Source: CAD feature listing. Evaluate the final solid. Frame: model axes, mm. A direction names the side the tool comes from. Round coordinates to 2 decimals unless told otherwise and drop trailing zeros. Order: outer loops, then holes, each group sorted by start corner. A loop starts at its lowest first (then second) coordinate and runs counter-clockwise, first axis right, second up. Notation, with made-up numbers: (56.25, 74.5) -> (68.25, 74.5) arc R15 ccw to (68.25, 86.5) -> close; hole circle Ø4 at (82.5, 8.25). An arc over 180 degrees is marked (long way). Answer as CSV lines item,"result".
from build123d import *

# Parameters (mm, degrees)
SKETCH_1_R            = 4.5
EXTRUDE_1_DEPTH       = 8
SKETCH_3_R            = 7.5
EXTRUDE_2_DEPTH       = 4
F_1_0MM_1_D           = 1
F_1_0MM_1_CSINK_D     = 6
F_1_0MM_1_CSINK_ANGLE = 90


with BuildPart() as part:
    # 草图1 → 凸台-拉伸1 (new body)
    with BuildSketch(Plane.XY):
        Circle(SKETCH_1_R)
    extrude(amount=EXTRUDE_1_DEPTH)

    # 草图3 → 凸台-拉伸2 (add)
    with BuildSketch(Plane.XY):
        Circle(SKETCH_3_R)
    extrude(amount=EXTRUDE_2_DEPTH)

    # Ø1.0mm 暗销孔1 (through all)
    with Locations(Plane(origin=(0, 0, 0), x_dir=(-1, 0, 0), z_dir=(0, 0, -1))):
        with Locations((0, 0)):
            CounterSinkHole(F_1_0MM_1_D / 2, F_1_0MM_1_CSINK_D / 2, counter_sink_angle=F_1_0MM_1_CSINK_ANGLE)


solid = part.part
1. Pin query (flat end, axial travel): pin 1 (4 mm diameter, centred on y = -4, z = 3, fed in from -X); pin 2 (4 mm diameter, centred on x = 5.5, y = 5.5, fed in from +Z); pin 3 (3 mm diameter, centred on y = 3, z = 6, fed in from +X). Return the tip coordinate at first contact, or that it passes through.
Results below:
pin 1,"x = -7.23"
pin 2,"z = 4"
pin 3,"x = 4.24"
2. Mould query, pull axis X, two halves, no side actions, for faces 3 (the conical face through (-0.71, -0.55, 2.1)), 4 (the cylindrical face through (-0.108, -0.488, 5.289)), 5 (the flat face through (3.2, 0.1, 0)), 6 (the cylindrical face through (-0.59, 4.46, 5.97)). Classes: released by +X, released by -X, zero draft, split by the parting line, or undercut.
Results below:
face 3,"undercut"
face 4,"undercut"
face 5,"zero draft"
face 6,"split by the parting line"
3. Section query A-A on x = 0. Return loops of the section in (y, z).
Results below:
outline,"(-7.5, 0) -> (-3, 0) -> (-0.5, 2.5) -> (-0.5, 8) -> (-4.5, 8) -> (-4.5, 4) -> (-7.5, 4) -> close; (0.5, 2.5) -> (3, 0) -> (7.5, 0) -> (7.5, 4) -> (4.5, 4) -> (4.5, 8) -> (0.5, 8) -> close"
4. Line query: L1, parallel to X at y = 0, z = 4.6; L2, parallel to X at y = 0.25, z = 7.25. Output: solid intervals per line, ascending. Write a range as [from, to].
Results below:
L1,"[-4.5, -0.5], [0.5, 4.5]"
L2,"[-4.49, -0.43], [0.43, 4.49]"
5. Section query D-D on z = 1. Return loops of the section in (x, y), and give its area (3 significant figures).
Results below:
outline,"circle Ø15 at (0, 0); hole circle Ø4 at (0, 0)"
area,"164 mm2"
6. Section query C-C on z = 6. Return loops of the section in (x, y), and give its area (3 significant figures).
Results below:
outline,"circle Ø9 at (0, 0); hole circle Ø1 at (0, 0)"
area,"62.8 mm2"
7. Reachability of faces 1 (the flat face through (0, -5, 4)), 2 (the cylindrical face through (-7.493, 0.33, 1.972)) from +Z, -Z, +X, -X, +Y, -Y: full face, straight path, thin tool, end or side. Return the list, or none.
Results below:
face 1,"+Z"
face 2,"+Z, -Z"
